Verification items for the finished model (mm, model axes). A direction names the side the tool comes from. Round coordinates to 2 decimals unless told otherwise and drop trailing zeros. Order: outer loops, then holes, each group sorted by start corner. A loop starts at its lowest first (then second) coordinate and runs counter-clockwise, first axis right, second up. Notation, with made-up numbers: M 25,4 L 42,4 A26 ccw 42,24 Z; hole C -10.75,54 d2. An arc over 180 degrees is marked long. Use CSV: the item, a comma, the result in double quotes. Start each with the question number.
Q1. Sectioned sample at D-D (x = -20). Enter the section's corners in (y, z).
Q2. Sectioned sample at C-C (y = -38.5). Enter the section's corners in (x, z), and give its area (3 significant figures).
Q3. Mould release check, pull along Y, two halves, no side actions. Record for faces 3 (the face through (0, -43.5, 1)), 4 (the face through (-21, 7.5, 1)), 5 (the face through (-11.5, 0.07, 0.99)), 6 (the face through (-16, -12, 2)): +Y half, -Y half, draft (parallel to the pull), parting line (faces both ways), or undercut.
Q4. Sectioned sample at B-B (z = 0.9). Enter the section's corners in (x, y), and give its area (3 significant figures).
Q5. Sectioned sample at A-A (y = 0). Enter the section's corners in (x, z).
Q6. Set-up check for faces 1 (the face through (-41, -13.6, 1)), 2 (the face through (5, -18, 1)): record each of +Z, -Z, +X, -X, +Y, -Y from which the full face is reachable in a straight line by a thin tool's end or side.
Q7. Gauge pin test, flat end, axial feed: pin 1 Ø1 at (y, z) = (-10.5, 1) entering from -X. Record the tip position at first contact, or that the pin passes through.
Q8. Scan lines: line 1 (Y direction, x = -0.5, z = 1.3); line 2 (Y direction, x = -32, z = 0.5); line 3 (Y direction, x = -35, z = 1.4). Record each from-to range of solid material in increasing order.
```python
from build123d import *

# Parameters (mm, degrees)
SKETCH_1_R          = 1.5
SKETCH_1_R_2        = 4.05
EXTRUDE_1_DEPTH     = 2
SKETCH_2_R          = 0.5
CUT_EXTRUDE_1_DEPTH = 10
FILLET_1_R          = 1


with BuildPart() as part:
    # 草图1 → 凸台-拉伸1 (new body)
    with BuildSketch(Plane.XY):
        Polygon((-47, -14.091283395), (-5, -43.5), (5, -43.5), (5, 7.5), (-47, 7.5), (-47, -7.4), (-34.9, -7.4), (-34.9, -13.6), (-47, -13.6), align=None)
        with Locations((0, -38.5)):
            Circle(SKETCH_1_R, mode=Mode.SUBTRACT)
        with Locations((0, -28.5)):
            Circle(SKETCH_1_R, mode=Mode.SUBTRACT)
        with Locations((-32, 0)):
            Circle(SKETCH_1_R, mode=Mode.SUBTRACT)
        with Locations((-20, 0)):
            Circle(SKETCH_1_R_2, mode=Mode.SUBTRACT)
        with Locations((-10, 0)):
            Circle(SKETCH_1_R, mode=Mode.SUBTRACT)
        Circle(SKETCH_1_R, mode=Mode.SUBTRACT)
    extrude(amount=EXTRUDE_1_DEPTH)

    # 草图2 → 切除-拉伸1 (cut)
    with BuildSketch(Plane(origin=(0, 0, 0), x_dir=(-1, 0, 0), z_dir=(0, 0, -1))):
        with Locations((34.9, -7.4)):
            Circle(SKETCH_2_R)
        with Locations((34.9, -13.6)):
            Circle(SKETCH_2_R)
    extrude(amount=-CUT_EXTRUDE_1_DEPTH, mode=Mode.SUBTRACT)

    # 圆角1
    fillet_1_edges = [part.edges().sort_by_distance(p)[0] for p in [
        (-47, -7.4, 1),
        (-47, 7.5, 1),
        (5, 7.5, 1),
        (5, -43.5, 1),
        (-5, -43.5, 1),
    ]]
    fillet(fillet_1_edges, radius=FILLET_1_R)


solid = part.part
```
Verdict:
1,outline,"M -33,0 L -4.05,0 L -4.05,2 L -33,2 Z; M 4.05,0 L 7.5,0 L 7.5,2 L 4.05,2 Z"
2,outline,"M -12.14,0 L -1.5,0 L -1.5,2 L -12.14,2 Z; M 1.5,0 L 5,0 L 5,2 L 1.5,2 Z"
2,area,"28.3 mm²"
3,face 3,"-Y half"
3,face 4,"+Y half"
3,face 5,"undercut"
3,face 6,"draft"
4,outline,"M -47,-14.09 L -5.26,-43.32 A1 ccw -4.68,-43.5 L 4,-43.5 A1 ccw 5,-42.5 L 5,6.5 A1 ccw 4,7.5 L -46,7.5 A1 ccw -47,6.5 L -47,-6.4 A1 ccw -46,-7.4 L -35.4,-7.4 A0.5 cw long -34.9,-7.9 L -34.9,-13.1 A0.5 cw long -35.4,-13.6 L -47,-13.6 Z; hole C -32,0 d3; hole C -20,0 d8.1; hole C -10,0 d3; hole C 0,-38.5 d3; hole C 0,-28.5 d3; hole C 0,0 d3"
4,area,"1,870 mm²"
5,outline,"M -47,0 L -33.5,0 L -33.5,2 L -47,2 Z; M -30.5,0 L -24.05,0 L -24.05,2 L -30.5,2 Z; M -15.95,0 L -11.5,0 L -11.5,2 L -15.95,2 Z; M -8.5,0 L -1.5,0 L -1.5,2 L -8.5,2 Z; M 1.5,0 L 5,0 L 5,2 L 1.5,2 Z"
6,face 1,"+Z, -Z, -X"
6,face 2,"+Z, -Z, +X, +Y, -Y"
7,pin 1,"stops at x = -34.9"
8,line 1,"y = -43.5 to -39.91, -37.09 to -29.91, -27.09 to -1.41, 1.41 to 7.5"
8,line 2,"y = -24.59 to -1.5, 1.5 to 7.5"
8,line 3,"y = -22.49 to -14.09, -6.91 to 7.5"
